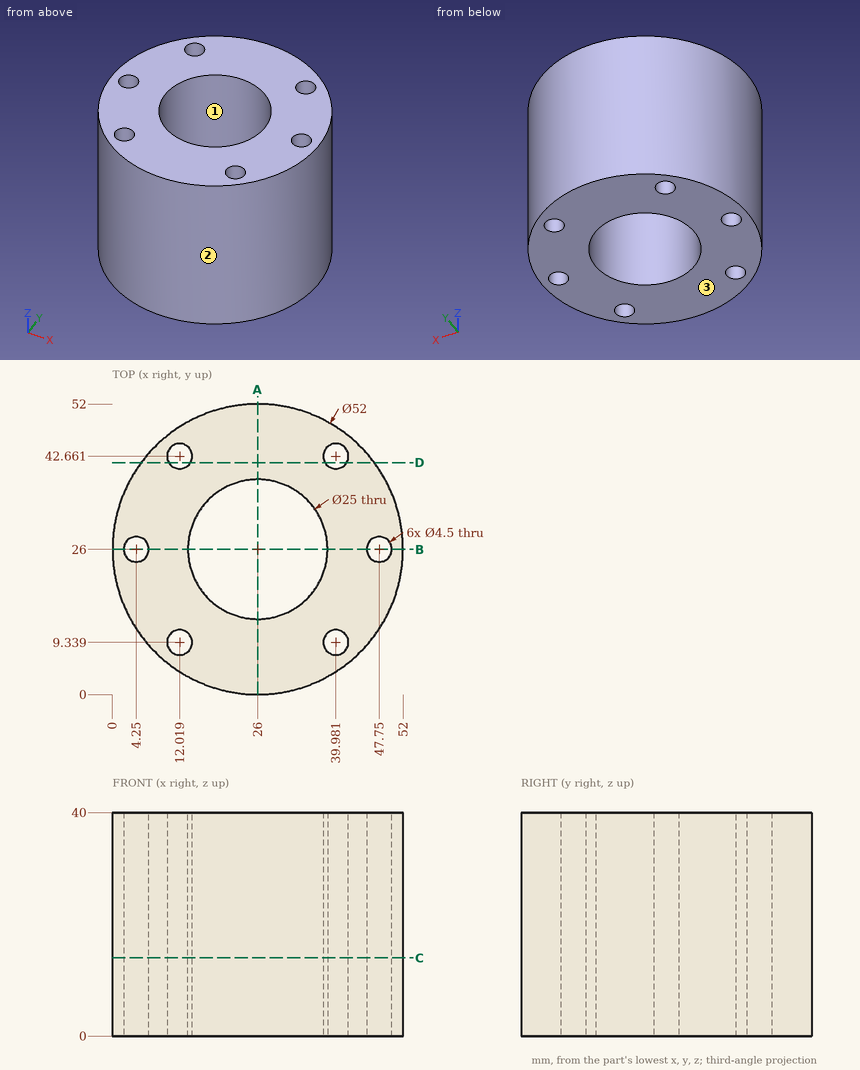
Job drawing, mm, ordinate dimensions from the low corner. One solid piece. Round coordinates to 2 decimals unless told otherwise and drop trailing zeros. Write each loop counter-clockwise with the first axis right and the second up, starting at its lowest first coordinate (ties: lowest second). Pieces come first, ordered by that corner, then holes. Notation, with made-up numbers: M 10.5,-23.75 L 34.5,-23.75 A22 ccw 34.5,-4.75 Z; hole C 74,9 d1. An arc over 180 degrees is marked long. Return JSON: item names as keys, results as strings. Group by question number.
(1) Saw through at D-D on y = 41.5. Write the cut outline in (x, z) (1 decimal).
(2) Saw through at B-B on y = 26. Write the cut outline in (x, z).
(3) Drill centre lines: probe 1 along X at (y, z) = (10.5, 29) (1 decimal); probe 2 along X at (y, z) = (28, 34) (1 decimal); probe 3 along X at (y, z) = (44, 32.5). Where is each one in solid material? Low to high.
(4) Two-plate mould, pull along Y, no slides. Class the marked faces 1, 2 and 3: +Y half, -Y half, draft (parallel to the pull), parting line (faces both ways), or undercut.
(5) Saw through at A-A on x = 26. Write the cut outline in (y, z).
(6) Saw through at C-C on z = 14. Write the cut outline in (x, y).
(7) Pin check, flat tips, straight feed: pin 1 Ø1.5 at (x, z) = (11.5, 6.5) entering from -Y; pin 2 Ø6 at (y, z) = (5.5, 26) entering from +X; pin 3 Ø1.5 at (x, z) = (25.5, 24) entering from -Y. Stop position of each tip, or through.
Returned:
{
 "1": {"outline": "M 5.1,0 L 10.1,0 L 10.1,40 L 5.1,40 Z; M 13.9,0 L 38.1,0 L 38.1,40 L 13.9,40 Z; M 41.9,0 L 46.9,0 L 46.9,40 L 41.9,40 Z"},
 "2": {"outline": "M 0,0 L 2,0 L 2,40 L 0,40 Z; M 6.5,0 L 13.5,0 L 13.5,40 L 6.5,40 Z; M 38.5,0 L 45.5,0 L 45.5,40 L 38.5,40 Z; M 50,0 L 52,0 L 52,40 L 50,40 Z"},
 "3": {"probe 1": "5.1 to 10.1, 13.9 to 38.1, 41.9 to 46.9", "probe 2": "0.1 to 3.2, 5.3 to 13.7, 38.3 to 46.7, 48.8 to 51.9", "probe 3": "7.24 to 10.21, 13.83 to 38.17, 41.79 to 44.76"},
 "4": {"face 1": "undercut", "face 2": "parting line", "face 3": "draft"},
 "5": {"outline": "M 0,0 L 13.5,0 L 13.5,40 L 0,40 Z; M 38.5,0 L 52,0 L 52,40 L 38.5,40 Z"},
 "6": {"outline": "C 26,26 d52; hole C 4.25,26 d4.5; hole C 12.02,9.34 d4.5; hole C 12.02,42.66 d4.5; hole C 26,26 d25; hole C 39.98,9.34 d4.5; hole C 39.98,42.66 d4.5; hole C 47.75,26 d4.5"},
 "7": {"pin 1": "y = 3.93", "pin 2": "x = 45.23", "pin 3": "y = 0"}
}
